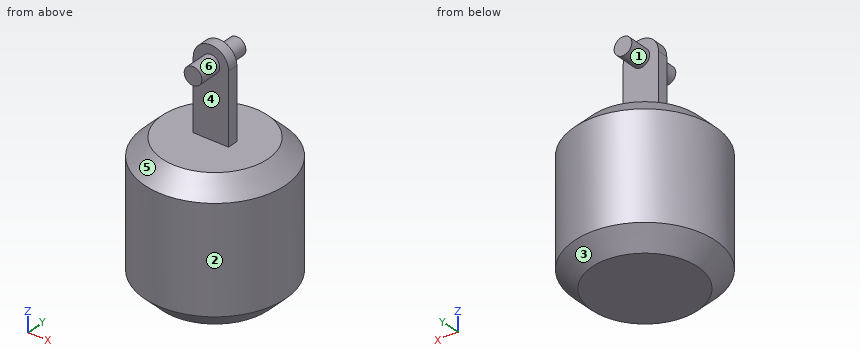
from build123d import *

# Parameters (mm, degrees)
F0_R     = 2.5
F1_DEPTH = 8
F3_DEPTH = 1.5
F4_R     = 20
F5_DEPTH = 39.84388
F6_SIZE  = 5


with BuildPart() as f1:
    # F0 (on Front) → F1 (new body, symmetric)
    with BuildSketch(Plane.XZ):
        Circle(F0_R)
    extrude(amount=F1_DEPTH, both=True)

    # F2 (on Front) → F3 (join, symmetric)
    with BuildSketch(Plane.XZ):
        with BuildLine():
            ThreePointArc((5, 0), (0, 5), (-5, 0))
            Line((-5, 0), (-5, -20))
            Line((-5, -20), (5, -20))
            Line((5, -20), (5, 0))
        make_face()
    extrude(amount=F3_DEPTH, both=True)

    # F4 (on face) → F5 (join)
    with BuildSketch(Plane(origin=(0, 0, -20), x_dir=(1, 0, 0), z_dir=(0, 0, -1))):
        Circle(F4_R)
    extrude(amount=F5_DEPTH)

    # F6
    f6_edges = [f1.edges().sort_by_distance(p)[0] for p in [
        (-20, 0, -20),
        (-20, 0, -59.84388),
    ]]
    chamfer(f6_edges, length=F6_SIZE)


solid = f1.part
For this review, take the finished solid that the model builds, in its own axes (mm). Face numbers are marked on the shaded views. A direction names the side the tool comes from. Give positions to 0.01 mm unless a question says otherwise; leave off trailing zeros. Order: outer loops, then holes, each group sorted by start corner. A loop starts at its lowest first (then second) coordinate and runs counter-clockwise, first axis right, second up. Notation, with made-up numbers: (26.5, 19.25) - (65.5, 19.25) arc R28 ccw to (65.5, 42.25) - close; hole circle Ø3 at (59.5, -21.75). An arc over 180 degrees is marked (long way). Answer as a JSON object with one key per item and string values. Group by question number.
Item 1: Wall thickness on line 1 along Z through (x, y) = (-12.5, 2); line 2 along X through (y, z) = (0, -2); line 3 along Y through (x, z) = (-1.5, -17): over which ranges is each line inside the solid? List them lowest first.
Item 2: Take a section at A-A on x = 0. Give the boundary of the cut face in (y, z), and give its area (3 significant figures).
Item 3: Draft analysis for pull direction Z (two halves, no side actions). For the marked faces 1, 2, 3 and 4, state which applies: pulls with the +Z half, pulls with the -Z half, needs draft (parallel to the pull), parting line crosses it, or undercut.
Item 4: Clearance check with flat-ended pins moving along their axes: pin 1 Ø9 at (x, y) = (7, -5) entering from +Z; pin 2 Ø8 at (x, z) = (-2, -6) entering from +Y; pin 3 Ø3.5 at (y, z) = (0.5, -6) entering from -X. State where each tip first meets the part, or that it passes through.
Item 5: Machinability: for the marked faces 5 and 6, which of the approach directions +Z, -Z, +X, -X, +Y, -Y give a long, thin tool a straight path to every point of the face, cutting with its end or side? Answer none if there is none.
Item 6: Take a section at B-B on y = 0. Give the boundary of the cut face in (x, z), and give its area (3 significant figures).
Item 7: Take a section at D-D on z = -12. Give the boundary of the cut face in (x, y), and give its area (3 significant figures).
Item 8: Take a section at C-C on z = -32. Give the boundary of the cut face in (x, y).
Reported:
{
 "1": {"line 1": "-59.84 to -20", "line 2": "-5 to 5", "line 3": "-1.5 to 1.5"},
 "2": {"outline": "(-20, -54.84) - (-15, -59.84) - (15, -59.84) - (20, -54.84) - (20, -25) - (15, -20) - (1.5, -20) - (1.5, -2.5) - (8, -2.5) - (8, 2.5) - (1.5, 2.5) - (1.5, 5) - (-1.5, 5) - (-1.5, 2.5) - (-8, 2.5) - (-8, -2.5) - (-1.5, -2.5) - (-1.5, -20) - (-15, -20) - (-20, -25) - close", "area": "1,680 mm^2"},
 "3": {"face 1": "undercut", "face 2": "needs draft", "face 3": "pulls with the -Z half", "face 4": "undercut"},
 "4": {"pin 1": "z = 2.76", "pin 2": "y = 8", "pin 3": "x = -5"},
 "5": {"face 5": "+Z", "face 6": "-Y"},
 "6": {"outline": "(-20, -54.84) - (-15, -59.84) - (15, -59.84) - (20, -54.84) - (20, -25) - (15, -20) - (5, -20) - (5, 0) arc R5 ccw to (-5, 0) - (-5, -20) - (-15, -20) - (-20, -25) - close", "area": "1,780 mm^2"},
 "7": {"outline": "(-5, -1.5) - (5, -1.5) - (5, 1.5) - (-5, 1.5) - close", "area": "30.0 mm^2"},
 "8": {"outline": "circle Ø40 at (0, 0)"}
}
